Can you work these out from the model? Positions are in its coordinate system, mm. A direction names the side the tool comes from. Give positions to 0.01 mm unless a question says otherwise; leave off trailing zeros. Write each loop counter-clockwise with the first axis right and the second up, starting at its lowest first coordinate (ties: lowest second). Pieces come first, ordered by that corner, then holes. Notation, with made-up numbers: (2, 6) - (33, 6) arc R24 ccw to (33, 22) - close; hole circle Ø5 at (-1.5, -13). An arc over 180 degrees is marked (long way). Use a Markdown table: item, result. Add a question column.
Autodesk Inventor part; units mm, degrees
ref_plane "YZ Plane" through (0, 0, 0) normal (1, 0, 0) x (0, 1, 0)
ref_plane "XZ Plane" through (0, 0, 0) normal (0, 1, 0) x (-1, 0, 0)
ref_plane "XY Plane" through (0, 0, 0) normal (0, 0, 1) x (1, 0, 0)
sketch "Boceto1" plane through (0, 0, 0) normal (0, 1, 0) x (-1, 0, 0)
  circle A0 centre (8.7689, 12.9363) radius 3
  circle A1 centre (8.7689, 12.9363) radius 5.11
  point P0 (0, 0)
  dimension "d0" = 6
  dimension "d1" = 10.22
extrude "Extrusión1" add sketch "Boceto1" along normal blind 20 contours A0
extrude "Extrusión2" add sketch "Boceto1" against normal blind 6 contours A0 | A1
sketch "Boceto2" plane through (-8.7689, -6, 12.9363) normal (0, -1, 0) x (1, 0, 0)
  line L0 (-2.5726, -1.4793) -> (-2.5674, 1.4883)
  line L1 (-2.5674, 1.4883) -> (0.0052, 2.9676)
  line L2 (0.0052, 2.9676) -> (2.5726, 1.4793)
  line L3 (2.5726, 1.4793) -> (2.5674, -1.4883)
  line L4 (2.5674, -1.4883) -> (-0.0052, -2.9676)
  line L5 (-0.0052, -2.9676) -> (-2.5726, -1.4793)
  point P0 (8.7689, -12.9363)
  point P1 (0, 0)
  dimension "d6" = 5.14
extrude "Extrusión3" cut sketch "Boceto2" against normal blind 3
thread "Rosca1"
chamfer "Chaflán1" distance 0.2 angle 45 1 edges at (-3.6589, -6, 12.9363) measured on face at (-12.1856, -6, 12.9393)
chamfer "Chaflán2" distance 0.2 angle 45 1 edges at (-5.7689, 20, 12.9363) measured on face at (-7.9784, 20, 13.0158)
properties part number "Tornillo allen cabeza cilindrica M6x20mm"
Q1. Suppose I cut it at A-A (y = -3.5). Please give me the cut outline in (x, z).
Q2. Suppose I cut it at B-B (y = 10). Please give me the cut outline in (x, z), and give its area (3 significant figures).
Q3. If we mould it in two halves opening along X, with no side actions, what happens to faces 1 (the flat face through (-9, 20, 13)), 2 (the cylindrical face through (-6.388, 9.761, 14.762)), 3 (the flat face through (-9, -3, 13))? For each: released by +X, released by -X, zero draft, split by the parting line, or undercut.
Q4. If I drill on probe 1 along Y at (x, z) = (-8.5, 15.25); probe 2 along Z at (x, y) = (-9.25, 16); probe 3 along Y at (x, z) = (-13, 12.75), over which ranges is the centre line in solid material (lowest first)? Write a range as [from, to].
Q5. I'm going to push flat-ended pins straight in: P1, Ø2, axis at x = -8.5, z = 11.5, coming from the -Y side; P2, Ø5, axis at y = 3, z = 17, coming from the +X side; P3, Ø1, axis at y = 7.5, z = 14, coming from the +X side. Where does each tip first touch, or does it pass through?
Q6. On a 3-axis mill with a long thin cutter (end or side, diameter ignored), from which of +Z, -Z, +X, -X, +Y, -Y can I reach the whole of each face in a straight line? I mean faces 4 (the flat face through (-11, -6, 11)), 5 (the flat face through (-7.5, -4.52, 15.17)), 6 (the flat face through (-11, 0, 10.7)). Say none if no direction works.
Derived:
| question | item | result |
|---|---|---|
| 1 | outline | circle Ø10.22 at (-8.77, 12.94); hole (-11.34, 11.46) - (-8.77, 9.97) - (-6.2, 11.45) - (-6.2, 14.42) - (-8.76, 15.9) - (-11.34, 14.42) - close |
| 2 | outline | circle Ø6 at (-8.77, 12.94) |
| 2 | area | 28.3 mm² |
| 3 | face 1 | zero draft |
| 3 | face 2 | split by the parting line |
| 3 | face 3 | undercut |
| 4 | probe 1 | [-3, 20] |
| 4 | probe 2 | [9.98, 15.9] |
| 4 | probe 3 | [-6, 0] |
| 5 | P1 | y = -3 |
| 5 | P2 | x = -6.21 |
| 5 | P3 | x = -5.82 |
| 6 | face 4 | +Z, -Z, +X, -X, -Y |
| 6 | face 5 | -Y |
| 6 | face 6 | +Y |
